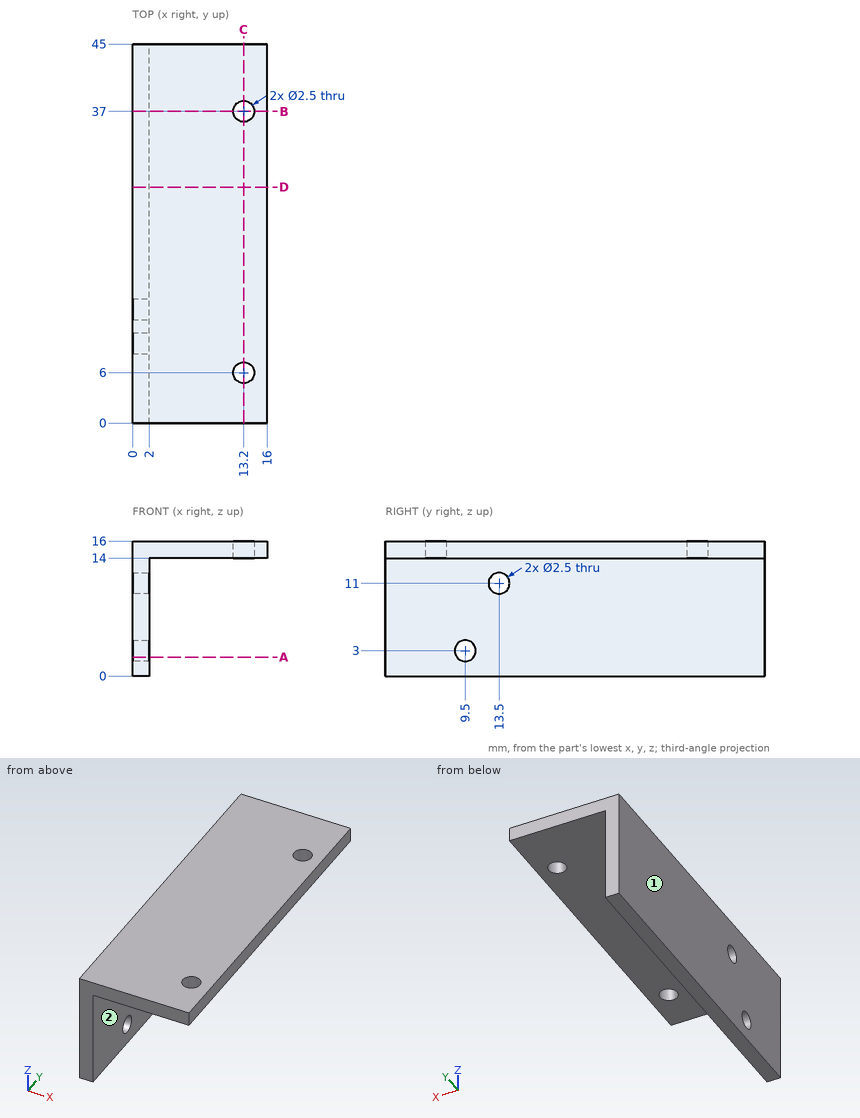
Study the drawing (mm; zero at the part's minimum x, y, z) and answer. A direction names the side the tool comes from. Coordinates: 2 decimals unless noted, no trailing zeros. Write each loop counter-clockwise with the first axis right and the second up, starting at its lowest first coordinate (ties: lowest second). Pieces come first, ordered by that corner, then holes. Notation, with made-up numbers: (-21, 75.5) - (11, 75.5) arc R21 cw to (11, 80.5) - close; hole circle Ø8 at (46.5, 11). An arc over 180 degrees is marked (long way). One line per item, written item: value.
1) Find section D-D (y = 28). Give the vertices of the cut face in (x, z), and give its area (3 significant figures).
Geometry check:
outline: (0, 0) - (2, 0) - (2, 14) - (16, 14) - (16, 16) - (0, 16) - close
area: 60.0 mm2
2) Each of these flat-tipped pins is pushed along its axis until it touches: pin 1 Ø4 at (y, z) = (28, 8) entering from +X; pin 2 Ø2 at (y, z) = (13.5, 11) entering from +X; pin 3 Ø7 at (x, y) = (8, 33.5) entering from -Z. Where does it stop, or does it pass through?
Geometry check:
pin 1: stops at x = 2
pin 2: passes through
pin 3: stops at z = 14
3) Find section B-B (y = 37). Give the vertices of the cut face in (x, z), and give its area (3 significant figures).
Geometry check:
outline: (0, 0) - (2, 0) - (2, 14) - (11.95, 14) - (11.95, 16) - (0, 16) - close; (14.45, 14) - (16, 14) - (16, 16) - (14.45, 16) - close
area: 55.0 mm2
4) Find section C-C (x = 13.2). Give the vertices of the cut face in (y, z).
Geometry check:
outline: (0, 14) - (4.75, 14) - (4.75, 16) - (0, 16) - close; (7.25, 14) - (35.75, 14) - (35.75, 16) - (7.25, 16) - close; (38.25, 14) - (45, 14) - (45, 16) - (38.25, 16) - close
5) Consider line 1 along Y through (x, z) = (13.2, 14.95); line 2 along Y through (x, z) = (1.45, 11); line 3 along X through (y, z) = (19.5, 12.75). Determine where each line is inside the solid, lowest interval first. Write a range as from..to.
Geometry check:
line 1: y = 0..4.75, 7.25..35.75, 38.25..45
line 2: y = 0..12.25, 14.75..45
line 3: x = 0..2
6) Find section A-A (z = 2.25). Give the vertices of the cut face in (x, y).
Geometry check:
outline: (0, 0) - (2, 0) - (2, 8.5) - (0, 8.5) - close; (0, 10.5) - (2, 10.5) - (2, 45) - (0, 45) - close
7) A tool of negligible diameter and unlimited length cuts with its end or side. For the marked faces 1 and 2, from which of +Z, -Z, +X, -X, +Y, -Y can it reach the whole face along a straight path? Write none if from no direction.
Geometry check:
face 1: +Z, -Z, -X, +Y, -Y
face 2: -Z, +X, +Y, -Y
